Part model, mm, in its own coordinate system. A direction names the side the tool comes from. Round coordinates to 2 decimals unless told otherwise and drop trailing zeros. Loops run counter-clockwise (first coordinate to the right, second up) from the corner with the lowest first, then second, coordinate; pieces in that order, holes last. Notation, with made-up numbers: (-38.75, -10) -> (1.25, -10) arc R11 ccw to (1.25, 3) -> close; hole circle Ø10 at (65, -22). An arc over 180 degrees is marked (long way). Use a Markdown table: item, result. Add a question column.
Item 1: Probe line 1 (Y direction, x = 11.25, z = 0); line 2 (Z direction, x = 19.25, y = 0). List the from-to ranges inside material, lowest first. Write a range as [from, to].
Item 2: Flat gauge pins, fed straight in: pin 1 (4 mm diameter, centred on x = 23.5, y = -3, fed in from -Z); pin 2 (1.5 mm diameter, centred on x = 12, z = 1, fed in from +Y); pin 3 (2.5 mm diameter, centred on y = 0, z = 0.5, fed in from -X). Where does each tip first touch, or does it go through?
Item 3: Cut at A-A, the plane z = 0. List the corners of the cut face in (x, y), plus the area to 3 significant figures.
Item 4: Cut at D-D, the plane z = -3. List the corners of the cut face in (x, y).
Item 5: Which spindle directions (+Z, -Z, +X, -X, +Y, -Y) get a long thin tool onto all of the face, cutting with end or side? Do faces 1 (the face through (12.68, 2.44, -0.54)), 2 (the face through (0, -2, 2)), 3 (the face through (13, -5, -2)). Say none if no direction does.
Item 6: Cut at B-B, the plane x = 11.75. List the corners of the cut face in (y, z).
Autodesk Inventor part; units mm, degrees
ref_plane "YZ Plane" through (0, 0, 0) normal (1, 0, 0) x (0, 1, 0)
ref_plane "XZ Plane" through (0, 0, 0) normal (0, 1, 0) x (-1, 0, 0)
ref_plane "XY Plane" through (0, 0, 0) normal (0, 0, 1) x (1, 0, 0)
sketch "Skizze1" plane through (0, 0, 0) normal (0, 1, 0) x (-1, 0, 0)
  line L0 (0, 0) -> (0, 4)
  line L1 (0, 4) -> (-10, 4)
  line L2 (-10, 4) -> (-10, 7)
  line L3 (-10, 7) -> (-13, 7)
  line L4 (-13, 7) -> (-13, 5)
  line L5 (-13, 5) -> (-23, 5)
  arc A0 (-23, 5) -> (-28, 0) centre (-23, 0) ccw
  line L6 (0, 0) -> (-28, 0)
  dimension "d0" = 3
  dimension "d1" = 10
  dimension "d2" = 15
  dimension "d3" = 14
  dimension "d4" = 8
  dimension "d5" = 10
revolve "Umdrehung1" add sketch "Skizze1" angle 360 about axis through (0, 0, 0) along (1, 0, 0)
thread "Gewinde1"
sketch "Skizze2" plane through (0, 0, 0) normal (-1, 0, 0) x (0, 0, 1)
  circle A0 centre (0, 0) radius 4
  point P0 (0, 0)
hole "Bohrung1" at (0, 0, 0) direction (1, 0, 0) diameter 5 depth 25
properties part number "1156"
A:
| question | item | result |
|---|---|---|
| 1 | line 1 | y = [-7, -2.5], [2.5, 7] |
| 1 | line 2 | z = [-5, -2.5], [2.5, 5] |
| 2 | pin 1 | stops at z = -4.89 |
| 2 | pin 2 | stops at y = 7 |
| 2 | pin 3 | stops at x = 25 |
| 3 | outline | (0, -4) -> (10, -4) -> (10, -7) -> (13, -7) -> (13, -5) -> (23, -5) arc R5 ccw to (23, 5) -> (13, 5) -> (13, 7) -> (10, 7) -> (10, 4) -> (0, 4) -> (0, 2.5) -> (25, 2.5) -> (25, -2.5) -> (0, -2.5) -> close |
| 3 | area | 136 mm^2 |
| 4 | outline | (0, -2.65) -> (10, -2.65) -> (10, -6.32) -> (13, -6.32) -> (13, -4) -> (23, -4) arc R4 ccw to (23, 4) -> (13, 4) -> (13, 6.32) -> (10, 6.32) -> (10, 2.65) -> (0, 2.65) -> close |
| 5 | face 1 | -X |
| 5 | face 2 | +Z, -Z, -X, +Y, -Y |
| 5 | face 3 | +X |
| 6 | outline | circle Ø14 at (0, 0); hole circle Ø5 at (0, 0) |
